Here's the drawing with two shaded views (mm, measured from the low corner). I have some questions. A direction names the side the tool comes from. Coordinates: 2 decimals unless noted, no trailing zeros. Loops run counter-clockwise (first coordinate to the right, second up) from the corner with the lowest first, then second, coordinate; pieces in that order, holes last. Notation, with made-up numbers: (30.5, 43.25) -> (78.5, 43.25) arc R26 cw to (78.5, 81.25) -> close; hole circle Ø3 at (49, 73). An arc over 180 degrees is marked (long way). Answer as a JSON object with one key per item and string values. Group by question number.
Q1. On a 3-axis mill with a long thin cutter (end or side, diameter ignored), from which of +Z, -Z, +X, -X, +Y, -Y can I reach the whole of each face in a straight line? I mean the marked faces 1, 2 and 3. Say none if no direction works.
Q2. I want a section at B-B on z = 80. Write out the boundary of the cut face in (x, y) (1 decimal).
Q3. Thinking about a two-plate mould opening in X: for the marked faces 4, 5, 6 and 7, which applies, released by +X, released by -X, zero draft, split by the parting line, or undercut?
Q4. I want a section at A-A on z = 25.5. Write out the boundary of the cut face in (x, y) (1 decimal).
Q5. I'm going to push flat-ended pins straight in: pin 1 (8 mm diameter, centred on y = 7, z = 46, fed in from -X); pin 2 (14 mm diameter, centred on x = 105, z = 90, fed in from -Y); pin 3 (14.5 mm diameter, centred on x = 10.51, z = 79.85, fed in from +Y); pin 4 (3 mm diameter, centred on y = 6, z = 47.5, fed in from +X). Where does each tip first touch, or does it pass through?
Q6. I need wall thicknesses on line 1 (X direction, y = 163.75, z = 79.85) (1 decimal); line 2 (X direction, y = 161, z = 124) (1 decimal); line 3 (Z direction, x = 74.5, y = 93). Which ranges of each line are inside material? Lowest first, please.
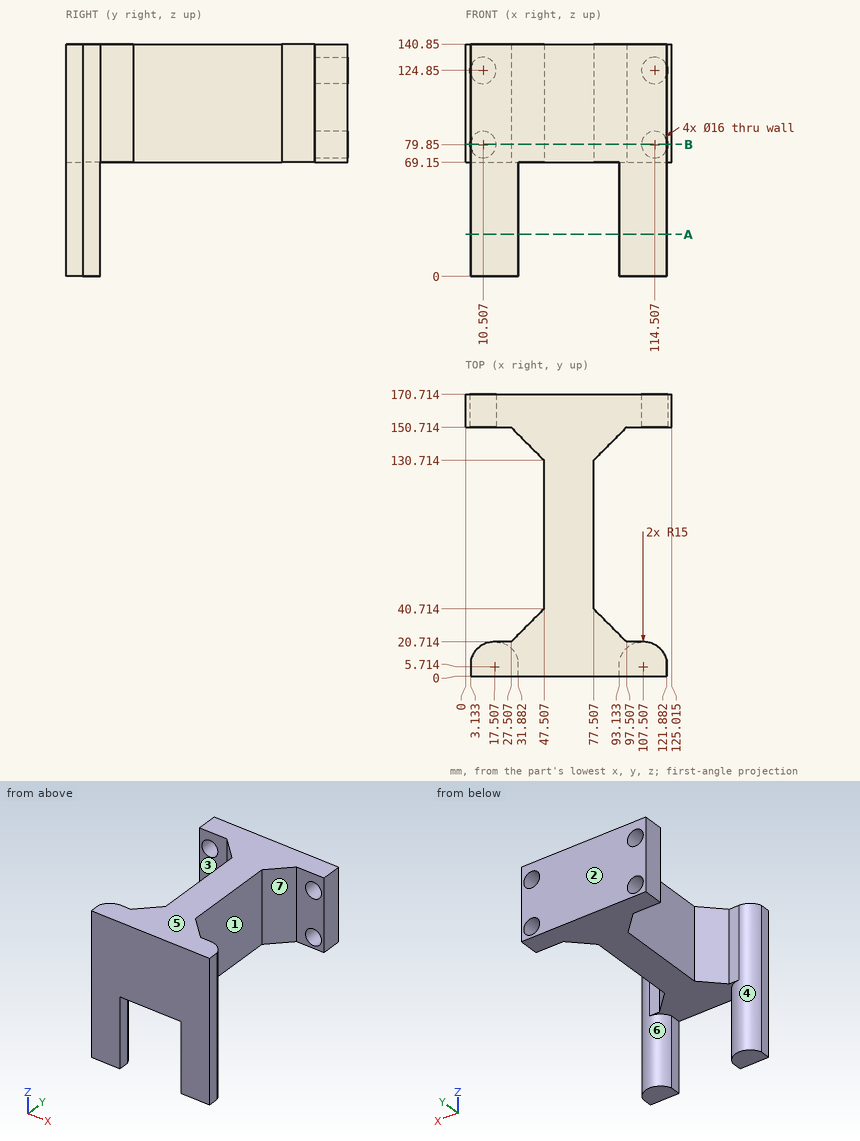
Result set:
{
 "1": {"face 1": "+Z, -Z, +X", "face 2": "+Z, -Z, +X, -X, +Y", "face 3": "+Z, -Z, -X"},
 "2": {"outline": "(0, 150.7) -> (2.5, 150.7) -> (2.5, 170.7) -> (0, 170.7) -> close; (3.1, 0) -> (121.9, 0) -> (121.9, 10) arc R15 ccw to (107.5, 20.7) -> (97.5, 20.7) -> (77.5, 40.7) -> (77.5, 130.7) -> (97.5, 150.7) -> (106.5, 150.7) -> (106.5, 170.7) -> (18.5, 170.7) -> (18.5, 150.7) -> (27.5, 150.7) -> (47.5, 130.7) -> (47.5, 40.7) -> (27.5, 20.7) -> (17.5, 20.7) arc R15 ccw to (3.1, 10) -> close; (122.5, 150.7) -> (125, 150.7) -> (125, 170.7) -> (122.5, 170.7) -> close"},
 "3": {"face 4": "undercut", "face 5": "zero draft", "face 6": "undercut", "face 7": "released by +X"},
 "4": {"outline": "(3.1, 0) -> (31.9, 0) -> (31.9, 10) arc R15 ccw to (3.1, 10) -> close; (93.1, 0) -> (121.9, 0) -> (121.9, 10) arc R15 ccw to (93.1, 10) -> close"},
 "5": {"pin 1": "stops at x = 3.13", "pin 2": "stops at y = 0", "pin 3": "stops at y = 20.71", "pin 4": "stops at x = 121.88"},
 "6": {"line 1": "x = 0 to 2.5, 18.5 to 106.5, 122.5 to 125", "line 2": "x = 0 to 2.6, 18.5 to 106.6, 122.5 to 125", "line 3": "z = 69.15 to 140.85"}
}
